```python
from build123d import *

# Parameters (mm, degrees)
BOX010_W     = 77
BOX010_H     = 2
BOX010_DEPTH = 2
BOX011_W     = 77
BOX011_H     = 2
BOX011_DEPTH = 2
BOX009_W     = 77
BOX009_H     = 2
BOX009_DEPTH = 2
BOX008_W     = 77
BOX008_H     = 10
BOX008_DEPTH = 2


with BuildPart() as cube010:
    # Box010 → Box010 (new body)
    with BuildSketch(Plane(origin=(5.5, 104, 12), x_dir=(1, 0, 0), z_dir=(0, 0, 1))):
        with Locations((38.5, 1)):
            Rectangle(BOX010_W, BOX010_H)
    extrude(amount=BOX010_DEPTH)


with BuildPart() as cube011:
    # Box011 → Box011 (new body)
    with BuildSketch(Plane(origin=(5.5, 108, 12), x_dir=(1, 0, 0), z_dir=(0, 0, 1))):
        with Locations((38.5, 1)):
            Rectangle(BOX011_W, BOX011_H)
    extrude(amount=BOX011_DEPTH)


with BuildPart() as cube009:
    # Box009 → Box009 (new body)
    with BuildSketch(Plane(origin=(5.5, 112, 12), x_dir=(1, 0, 0), z_dir=(0, 0, 1))):
        with Locations((38.5, 1)):
            Rectangle(BOX009_W, BOX009_H)
    extrude(amount=BOX009_DEPTH)


with BuildPart() as fusion:
    # Box008 → Box008 (new body)
    with BuildSketch(Plane(origin=(5.5, 104, 10), x_dir=(1, 0, 0), z_dir=(0, 0, 1))):
        with Locations((38.5, 5)):
            Rectangle(BOX008_W, BOX008_H)
    extrude(amount=BOX008_DEPTH)

    # Fusion: union Cube010, Cube011, Cube009
    add(cube010.part)
    add(cube011.part)
    add(cube009.part)


with BuildPart() as fusion_1:
    # Fusion placement: moved
    add(fusion.part.moved(Location((0, -100, 0))))


solid = fusion_1.part
```
Here's how the part is built. I have some questions about the finished solid (model axes, mm). A direction names the side the tool comes from. Give positions to 0.01 mm unless a question says otherwise; leave off trailing zeros. Write each loop counter-clockwise with the first axis right and the second up, starting at its lowest first coordinate (ties: lowest second). Pieces come first, ordered by that corner, then holes. Notation, with made-up numbers: (0.5, 57.25) -> (11.5, 57.25) arc R13 cw to (11.5, 71.25) -> close; hole circle Ø6 at (53.25, 88.25). An arc over 180 degrees is marked (long way). Write each question's results on one line, items separated by ' | '.
Item 1: If I drill on L1, parallel to Y at x = 64, z = 12.5; L2, parallel to Z at x = 68.5, y = 11.75, over which ranges is the centre line in solid material (lowest first)?
Output:
L1: y = 4 to 6, 8 to 10, 12 to 14 | L2: z = 10 to 12
Item 2: For pin 1 Ø0.6 at (x, y) = (59, 7) entering from +Z, with a flat end and sliding along its axis, tell me the tip position at first contact or that it passes through.
Output:
pin 1: stops at z = 12
Item 3: Suppose I cut it at B-B on y = 11. Write out the boundary of the cut face in (x, z).
Output:
outline: (5.5, 10) -> (82.5, 10) -> (82.5, 12) -> (5.5, 12) -> close
Item 4: Suppose I cut it at A-A on x = 56. Write out the boundary of the cut face in (y, z).
Output:
outline: (4, 10) -> (14, 10) -> (14, 14) -> (12, 14) -> (12, 12) -> (10, 12) -> (10, 14) -> (8, 14) -> (8, 12) -> (6, 12) -> (6, 14) -> (4, 14) -> close
Item 5: On a 3-axis mill with a long thin cutter (end or side, diameter ignored), from which of +Z, -Z, +X, -X, +Y, -Y can I reach the whole of each face in a straight line? I mean faces 4 (the face through (43, 8, 13)), 5 (the face through (43, 5, 14)). Say none if no direction works.
Output:
face 4: +Z, +X, -X | face 5: +Z, +X, -X, +Y, -Y
Item 6: We'd pull the mould along Y, two halves only. Please class faces 1 (the face through (43, 9, 10)), 2 (the face through (43, 4, 12)), 3 (the face through (43, 6, 13)): pulls with the +Y half, pulls with the -Y half, needs draft (parallel to the pull), parting line crosses it, or undercut.
Output:
face 1: needs draft | face 2: pulls with the -Y half | face 3: undercut
